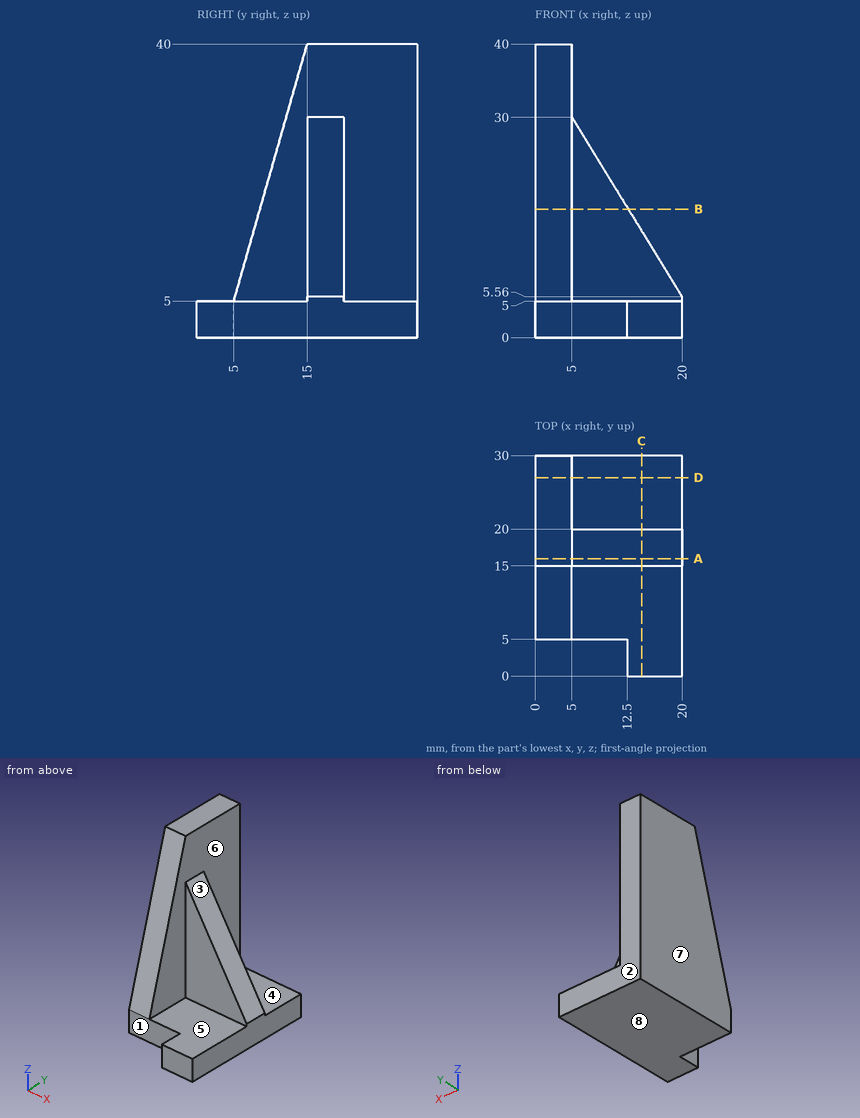
Source: three-view drawing plus pictorial views. Frame: mm from the lowest corner of the part. A direction names the side the tool comes from. Round coordinates to 2 decimals unless told otherwise and drop trailing zeros. Write each loop counter-clockwise with the first axis right and the second up, starting at its lowest first coordinate (ties: lowest second). Pieces come first, ordered by that corner, then holes. Notation, with made-up numbers: (-12.5, 82) -> (4.5, 82) arc R36 ccw to (4.5, 118) -> close; hole circle Ø3 at (1, -22.75). An arc over 180 degrees is marked (long way). Return JSON: item names as keys, results as strings.
Q1. First-contact query: pin 1 Ø7.5 at (x, z) = (14, 19.5) entering from +Y; pin 2 Ø3 at (x, z) = (18, 6) entering from +Y; pin 3 Ø7.5 at (y, z) = (23.5, 23) entering from +X; pin 4 Ø8 at (x, y) = (16, 26) entering from +Z. Flat tips, straight axial feed; report the tip coordinate or a pass-through.
From the geometry:
{"pin 1": "y = 20", "pin 2": "y = 30", "pin 3": "x = 10.12", "pin 4": "z = 5"}
Q2. Section C-C on x = 14.5. Return the cut outline in (y, z), and give its area (3 significant figures).
From the geometry:
{"outline": "(0, 0) -> (30, 0) -> (30, 5) -> (20, 5) -> (20, 14.52) -> (15, 14.52) -> (15, 5) -> (0, 5) -> close", "area": "198 mm2"}
Q3. Set-up query: the marked faces 4, 5, 6, 7 and 8. Return all of +Z, -Z, +X, -X, +Y, -Y with unobstructed straight access to the full face (end or side cutting, diameter ignored); none if empty.
From the geometry:
{"face 4": "+Z, +X, +Y", "face 5": "+Z, +X, -Y", "face 6": "+Z, +X", "face 7": "+Z, -Z, -X, +Y, -Y", "face 8": "-Z, +X, -X, +Y, -Y"}
Q4. Section A-A on y = 16. Return the cut outline in (x, z).
From the geometry:
{"outline": "(0, 0) -> (20, 0) -> (20, 5.56) -> (5, 30) -> (5, 40) -> (0, 40) -> close"}
Q5. Ray query, line 1 (Z direction, x = 12, y = 9.5); line 2 (Y direction, x = 10.75, z = 18). Return the intervals inside material, ascending.
From the geometry:
{"line 1": "0 to 5", "line 2": "15 to 20"}
Q6. Section D-D on y = 27. Return the cut outline in (x, z).
From the geometry:
{"outline": "(0, 0) -> (20, 0) -> (20, 5) -> (5, 5) -> (5, 40) -> (0, 40) -> close"}
Q7. Mould query, pull axis Y, two halves, no side actions, for the marked faces 1, 2 and 3. Classes: +Y half, -Y half, draft (parallel to the pull), parting line (faces both ways), or undercut.
From the geometry:
{"face 1": "-Y half", "face 2": "+Y half", "face 3": "draft"}
Q8. Section B-B on z = 17.5. Return the cut outline in (x, y).
From the geometry:
{"outline": "(0, 8.57) -> (5, 8.57) -> (5, 15) -> (12.67, 15) -> (12.67, 20) -> (5, 20) -> (5, 30) -> (0, 30) -> close"}
